Design review of the part built by this model. Coordinates are the model's own, in mm. A direction names the side the tool comes from. Give positions to 0.01 mm unless a question says otherwise; leave off trailing zeros. Loops run counter-clockwise (first coordinate to the right, second up) from the corner with the lowest first, then second, coordinate; pieces in that order, holes last. Notation, with made-up numbers: (13.25, 44) -> (53.25, 44) arc R27 cw to (53.25, 81) -> close; hole circle Ø7 at (43.25, 57). An arc over 180 degrees is marked (long way). Answer in a Markdown table with one row per item. Add a question column.
(1) Draft analysis for pull direction Y (two halves, no side actions). For faces 3 (the cylindrical face through (14.86, 4.73, 0.78)), 4 (the cylindrical face through (69.17, 41.273, 0.783)), 5 (the flat face through (0, 14, 1)), state which applies: +Y half, -Y half, draft (parallel to the pull), parting line (faces both ways), or undercut.
(2) For faces 1 (the flat face through (40, 9.271, 1)), 2 (the cylindrical face through (0.724, 0.764, 0.805)), list the 3-axis set-ups (+Z, -Z, +X, -X, +Y, -Y) from which the entire face can be reached by the end or side of a thin tool; tool diameter is ignored.
(3) Consider section B-B on x = 71. Write out the cut boundary in (y, z).
(4) Consider section A-A on y = 15.5. Write out the cut boundary in (x, z), then the cut area to 3 significant figures.
(5) Consider section D-D on x = 37. Write out the cut boundary in (y, z).
(6) Consider section C-C on z = 0.35. Count the separate pieces of the cut face and the enclosed holes in it, then the cut area to 3 significant figures.
(7) For pin 1 (0.5 mm diameter, centred on x = 48, z = 0.5, fed in from +Y), flat-tipped, find the tip position at first contact; note if it passes through.
(8) For line 1 (X direction, y = 19, z = 1.3); line 2 (Y direction, x = 9.5, z = 1.35), list the stretches that pass through material, from the lowest coordinate up.
from build123d import *

# Parameters (mm, degrees)
SKETCH1_R           = 2.159
SKETCH1_R_2         = 3.81
BOSS_EXTRUDE1_DEPTH = 1.5875
FILLET1_R           = 2.54


with BuildPart() as part:
    # Sketch1 → Boss-Extrude1 (new body)
    with BuildSketch(Plane.XY):
        with BuildLine():
            Line((0, 25.4), (0, 0))
            Line((0, 0), (78.486, 0))
            Line((78.486, 0), (78.486, 31.75))
            ThreePointArc((78.486, 31.75), (68.961, 41.275), (59.436, 31.75))
            Line((59.436, 31.75), (59.436, 9.271))
            Line((59.436, 9.271), (19.05, 9.271))
            Line((19.05, 9.271), (19.05, 25.4))
            ThreePointArc((19.05, 25.4), (9.525, 34.925), (0, 25.4))
        make_face()
        with Locations((17.018, 4.6355)):
            Circle(SKETCH1_R, mode=Mode.SUBTRACT)
        with Locations((61.468, 4.6355)):
            Circle(SKETCH1_R, mode=Mode.SUBTRACT)
        with Locations((9.525, 25.4)):
            Circle(SKETCH1_R_2, mode=Mode.SUBTRACT)
        with Locations((68.961, 31.75)):
            Circle(SKETCH1_R_2, mode=Mode.SUBTRACT)
    extrude(amount=BOSS_EXTRUDE1_DEPTH)

    # Fillet1
    fillet1_edges = [part.edges().sort_by_distance(p)[0] for p in [
        (78.486, 0, 0.79375),
        (0, 0, 0.79375),
    ]]
    fillet(fillet1_edges, radius=FILLET1_R)


solid = part.part
Values follow:
| question | item | result |
|---|---|---|
| 1 | face 3 | undercut |
| 1 | face 4 | +Y half |
| 1 | face 5 | draft |
| 2 | face 1 | +Z, -Z, +Y |
| 2 | face 2 | +Z, -Z, -X, -Y |
| 3 | outline | (0, 0) -> (28.53, 0) -> (28.53, 1.59) -> (0, 1.59) -> close; (34.97, 0) -> (41.05, 0) -> (41.05, 1.59) -> (34.97, 1.59) -> close |
| 4 | outline | (0, 0) -> (19.05, 0) -> (19.05, 1.59) -> (0, 1.59) -> close; (59.44, 0) -> (78.49, 0) -> (78.49, 1.59) -> (59.44, 1.59) -> close |
| 4 | area | 60.5 mm2 |
| 5 | outline | (0, 0) -> (9.27, 0) -> (9.27, 1.59) -> (0, 1.59) -> close |
| 6 | separate pieces | 1 |
| 6 | enclosed holes | 4 |
| 6 | area | 1,620 mm2 |
| 7 | pin 1 | y = 9.27 |
| 8 | line 1 | 0 to 19.05, 59.44 to 78.49 |
| 8 | line 2 | 0 to 21.59, 29.21 to 34.92 |
